Design review of the part built by this model. Coordinates are the model's own, in mm. A direction names the side the tool comes from. Round coordinates to 2 decimals unless told otherwise and drop trailing zeros. Loops run counter-clockwise (first coordinate to the right, second up) from the corner with the lowest first, then second, coordinate; pieces in that order, holes last. Notation, with made-up numbers: (46.5, 69.5) - (50.5, 69.5) arc R27 cw to (50.5, 102.5) - close; hole circle Ø7 at (11, -21). An arc over 180 degrees is marked (long way). Use one line per item in the form item = value. Start each with the question number.
(1) The part is to be moulded in two halves that separate along X. For faces 5 (the flat face through (481.2, 623.53, -282.33)), 6 (the cylindrical face through (240.298, 24.65, 763.057)), 7 (the flat face through (544, 650, 311)), say which applies: released by +X, released by -X, zero draft, split by the parting line, or undercut.
(2) We need section C-C, the plane y = 461. Write out the cut boundary in (x, z), then the cut area to 3 significant figures.
(3) Machinability: for faces 1 (the flat face through (481, 596.306, 287)), 2 (the flat face through (650, 629, -37.5)), 3 (the flat face through (4, 624, 557.897)), 4 (the flat face through (-4, 650, -610)), which of the approach directions +Z, -Z, +X, -X, +Y, -Y give a long, thin tool a straight path to every point of the face, cutting with its end or side? Answer none if there is none.
(4) We need section B-B, the plane z = 0. Write out the cut boundary in (x, y), then the cut area to 3 significant figures.
(5) Wall thickness on probe 1 along X at (y, z) = (33, 0); probe 2 along X at (y, z) = (314.5, 464); probe 3 along Z at (x, y) = (583, 243.5): over which ranges is each line inside the solid? List them lowest first. Write a range as [from, to].
(6) We need section D-D, the plane y = 125.5. Write out the cut boundary in (x, z), then the cut area to 3 significant figures.
(7) We need section A-A, the plane x = 0. Write out the cut boundary in (y, z).
(8) For pin 1 (2 mm diameter, centred on x = -546.5, y = 523, fed in from -Z); pin 2 (4 mm diameter, centred on x = -517, y = 294.5, fed in from -Z); pin 3 (12 mm diameter, centred on x = 588, y = 428, fed in from -Z), all flat-tipped, find the tip position at first contact; note any pin that passes through.
from build123d import *

# Parameters (mm, degrees)
SKETCH1_R           = 800
SKETCH1_R_2         = 750
BOSS_EXTRUDE1_DEPTH = 50
SKETCH15_R          = 694.203811575
BOSS_EXTRUDE2_DEPTH = 53.694202
SKETCH18_W          = 70.63704417
SKETCH18_H          = 75
CUT_EXTRUDE4_DEPTH  = 130
CIRPATTERN1_COUNT   = 6


with BuildPart() as part:
    # Sketch1 → Boss-Extrude1 (new body)
    with BuildSketch(Plane(origin=(0, 0, 0), x_dir=(1, 0, 0), z_dir=(0, 1, 0))):
        with Locations(Location((0, 0, 0), (0, 0, 270))):
            Circle(SKETCH1_R)
        with Locations(Location((0, 0, 0), (0, 0, 270))):
            Circle(SKETCH1_R_2, mode=Mode.SUBTRACT)
    extrude(amount=BOSS_EXTRUDE1_DEPTH)

    # Sketch14 → Revolve1 (revolve)
    with BuildSketch(Plane(origin=(0, 0, 0), x_dir=(0, 0, -1), z_dir=(1, 0, 0)), mode=Mode.PRIVATE) as revolve1_sk:
        Polygon((-644.203811575, 650), (-750, 50), (-800, 50), (-694.203811575, 650), align=None)
    revolve(revolve1_sk.sketch.rotate(Axis((0, 0, 0), (0, 1, 0)), 180), axis=Axis((0, 0, 0), (0, 1, 0)))

    # Sketch15 → Boss-Extrude2 (add)
    with BuildSketch(Plane(origin=(0, 650, 0), x_dir=(1, 0, 0), z_dir=(0, 1, 0))):
        Circle(SKETCH15_R)
        Polygon((278.800635598, 557.896866039), (343.752540882, 520.396866039), (622.55317648, 37.5), (622.55317648, -37.5), (343.752540882, -520.396866039), (278.800635598, -557.896866039), (-278.800635598, -557.896866039), (-343.752540882, -520.396866039), (-622.55317648, -37.5), (-622.55317648, 37.5), (-343.752540882, 520.396866039), (-278.800635598, 557.896866039), align=None, mode=Mode.SUBTRACT)
    extrude(amount=-BOSS_EXTRUDE2_DEPTH)

    # Sketch18 → Cut-Extrude4 (cut, along a direction that is not the sketch's normal)
    with BuildSketch(Plane(origin=(0, 650, 0), x_dir=(1, 0, 0), z_dir=(0, 1, 0))):
        with Locations((657.871698565, 0)):
            Rectangle(SKETCH18_W, SKETCH18_H)
    cut_extrude4 = extrude(amount=-CUT_EXTRUDE4_DEPTH, dir=(0.7961076341406244, 0.6051550502664734, 0), mode=Mode.SUBTRACT)

    # CirPattern1: Cut-Extrude4 ×6 about axis
    cirpattern1_axis = Axis((0, 0, 0), (0, 1, 0))
    for i in range(1, CIRPATTERN1_COUNT):
        add(cut_extrude4.rotate(cirpattern1_axis, i * 360 / CIRPATTERN1_COUNT), mode=Mode.SUBTRACT)


solid = part.part
Data:
q1.face_5 = undercut
q1.face_6 = split by the parting line
q1.face_7 = zero draft
q2.outline = circle Ø1455.06 at (0, 0); hole circle Ø1355.06 at (0, 0)
q2.area = 221,000 mm^2
q3.face_1 = -Y
q3.face_2 = +Y
q3.face_3 = +Y, -Y
q3.face_4 = +Z, -Z, +X, -X, +Y
q4.outline = (-800, 0) - (-750, 0) - (-750, 50) - (-653.67, 596.31) - (-622.55, 596.31) - (-693.19, 650) - (-694.2, 650) - (-800, 50) - close; (622.55, 596.31) - (653.67, 596.31) - (750, 50) - (750, 0) - (800, 0) - (800, 50) - (694.2, 650) - (693.19, 650) - close
q4.area = 64,000 mm^2
q5.probe_1 = [-800, -750], [750, 800]
q5.probe_2 = [-593.51, -528.6], [528.6, 593.51]
q5.probe_3 = [-496.67, -415.45], [415.45, 496.67]
q6.outline = circle Ø1573.37 at (0, 0); hole circle Ø1473.37 at (0, 0)
q6.area = 239,000 mm^2
q7.outline = (0, -800) - (50, -800) - (650, -694.2) - (650, -557.9) - (596.31, -557.9) - (596.31, -653.67) - (50, -750) - (0, -750) - close; (0, 750) - (50, 750) - (596.31, 653.67) - (596.31, 557.9) - (650, 557.9) - (650, 694.2) - (50, 800) - (0, 800) - close
q8.pin_1 = -464.73
q8.pin_2 = -554.73
q8.pin_3 = -446.37
